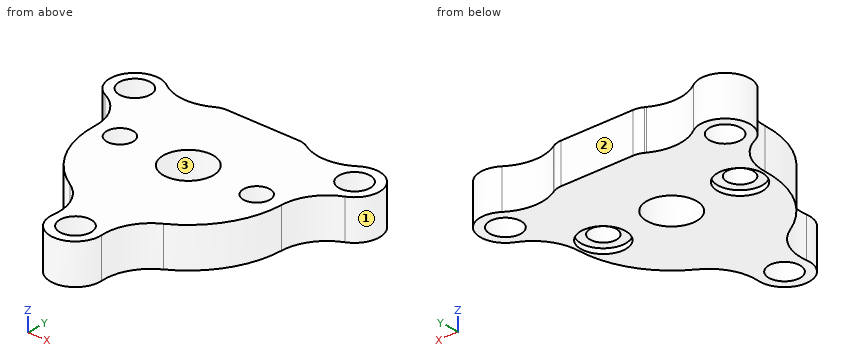
Autodesk Inventor part; units mm, degrees
ref_plane "YZ Plane" through (0, 0, 0) normal (1, 0, 0) x (0, 1, 0)
ref_plane "XZ Plane" through (0, 0, 0) normal (0, 1, 0) x (-1, 0, 0)
ref_plane "XY Plane" through (0, 0, 0) normal (0, 0, 1) x (1, 0, 0)
sketch "Sketch1" plane through (0, 0, 0) normal (0, 0, 1) x (1, 0, 0)
  circle A0 centre (0, 0) radius 20.7359 construction
  line L0 (0, 0) -> (-17.9578, 10.368) construction
  arc A1 (-19.6042, 6.7568) -> (-15.6537, 13.5993) centre (-17.9578, 10.368) ccw construction
  arc A2 (-7.603, 13.208) -> (-15.24, -0.0196) centre (0, 0) ccw construction
  arc A3 (-15.24, -0.0196) -> (-19.6042, 6.7568) centre (-22.698, -0.0292) ccw
  arc A4 (-15.6537, 13.5993) -> (-7.603, 13.208) centre (-11.3237, 19.6716) ccw
  line L1 (0, 0) -> (-20.7359, 0) construction
  arc A5 (-15.6537, 13.5993) -> (-19.6042, 6.7568) centre (-17.9578, 10.368) ccw
  arc A6 (-15.24, -0.0196) -> (-7.637, -13.1884) centre (0, 0) ccw
  arc A7 (7.637, -13.1884) -> (3.9505, -20.3561) centre (11.3743, -19.6424) ccw
  arc A8 (-3.9505, -20.3561) -> (-7.637, -13.1884) centre (-11.3743, -19.6424) ccw
  arc A9 (-3.9505, -20.3561) -> (3.9505, -20.3561) centre (0, -20.7359) ccw
  arc A10 (7.603, 13.208) -> (15.6537, 13.5993) centre (11.3237, 19.6716) ccw
  arc A11 (19.6042, 6.7568) -> (15.24, -0.0196) centre (22.698, -0.0292) ccw
  arc A12 (19.6042, 6.7568) -> (15.6537, 13.5993) centre (17.9578, 10.368) ccw
  arc A13 (7.603, 13.208) -> (6.643, 13.716) centre (0, 0) ccw
  arc A14 (7.637, -13.1884) -> (15.24, -0.0196) centre (0, 0) ccw
  arc A15 (-7.637, -13.1884) -> (7.637, -13.1884) centre (0, 0) ccw construction
  arc A16 (15.24, -0.0196) -> (7.603, 13.208) centre (0, 0) ccw construction
  circle A17 centre (0, 0) radius 3.9688
  circle A18 centre (0, 0) radius 11.176 construction
  line L2 (0, -20.7359) -> (0, 0) construction
  line L3 (0, 0) -> (11.176, 0) construction
  line L4 (-6.643, 13.716) -> (6.643, 13.716)
  arc A19 (-6.643, 13.716) -> (-7.603, 13.208) centre (0, 0) ccw
  arc A20 (6.643, 13.716) -> (-6.643, 13.716) centre (0, 0) ccw construction
  point P0 (-11.176, 0)
  dimension "d0" = 41.4719
  dimension "d3" = 7.9375
  dimension "d5" = 30
  dimension "d9" = 360
  dimension "d20" = 7.9375
  dimension "d21" = 22.352
  dimension "d22" = 15.24
  dimension "d23" = 13.716
extrude "Extrusion1" add sketch "Sketch1" along normal blind 6.35
hole "Hole1" at (-17.9578, 10.368, 0) at (17.9578, 10.368, 0) at (0, -20.7359, 0) direction (0, 0, 1) diameter 4.9784 end through all
hole "Hole2" at (-11.176, 0, 0) at (11.176, 0, 0) direction (0, 0, 1) diameter 4.2164 end through all
fillet "Fillet1" radius 3.175 2 edges at (-6.643, 13.716, 3.175) (6.643, 13.716, 3.175)
sketch "Sketch2" plane through (0, 0, 0) normal (0, 0, -1) x (-1, 0, 0)
  circle A0 centre (11.176, 0) radius 2.1082
  circle A1 centre (-11.176, 0) radius 2.1082
  circle A2 centre (-11.176, 0) radius 3.5719
  circle A3 centre (11.176, 0) radius 3.5719
  dimension "d32" = 7.1437
  dimension "d33" = 7.1437
extrude "Extrusion2" cut sketch "Sketch2" against normal blind 0.7937
properties part number "Pnuematic Plate" material "Aluminum 6061"
Design review of the part built by this model. Coordinates are the model's own, in mm. Face numbers are marked on the shaded views. Give positions to 0.01 mm unless a question says otherwise; leave off trailing zeros. Order: outer loops, then holes, each group sorted by start corner. A loop starts at its lowest first (then second) coordinate and runs counter-clockwise, first axis right, second up.
1. Add section D-D, the plane x = 14. State the section outline as (y, z) points.
Solution:
outline: (-6.02, 0) - (-2.19, 0) - (-2.19, 0.79) - (2.19, 0.79) - (2.19, 0) - (12.71, 0) - (12.71, 6.35) - (-6.02, 6.35) - close
2. Mouldability with a two-part tool opening along Y and no side actions: class the marked faces 1, 2 and 3 as +Y half, -Y half, draft (parallel to the pull), parting line (faces both ways), or undercut.
Solution:
face 1: parting line
face 2: +Y half
face 3: undercut
3. For pin 1 Ø5.5 at (x, y) = (11.176, 0) entering from +Z; pin 2 Ø1.9 at (x, z) = (-1, 4) entering from +Y; pin 3 Ø1.5 at (y, z) = (-20.5, 2) entering from -X; pin 4 Ø3 at (y, z) = (-1, 2.5) entering from +X, all flat-tipped, find the tip position at first contact; note any pin that passes through.
Solution:
pin 1: stops at z = 6.35
pin 2: stops at y = 13.72
pin 3: stops at x = -3.97
pin 4: stops at x = 15.26
4. Add section C-C, the plane y = -4.5. State the section outline as (x, z) points.
Solution:
outline: (-14.56, 0) - (14.56, 0) - (14.56, 6.35) - (-14.56, 6.35) - close
5. To check wall thickness, follow L1, parallel to Y at x = 0.5, z = 2; L2, parallel to Y at x = 11, z = 5; L3, parallel to Y at x = -13, z = 0.75. State the ranges of each line that lie inside material, in increasing order.
Solution:
L1: y = -24.67 to -23.17, -18.3 to -3.94, 3.94 to 13.72
L2: y = -10.55 to -2.1, 2.1 to 12.22
L3: y = -7.95 to -3.07, 3.07 to 12.4
6. Add section A-A, the plane x = 0. State the section outline as (y, z) points.
Solution:
outline: (-24.7, 0) - (-23.23, 0) - (-23.23, 6.35) - (-24.7, 6.35) - close; (-18.25, 0) - (-3.97, 0) - (-3.97, 6.35) - (-18.25, 6.35) - close; (3.97, 0) - (13.72, 0) - (13.72, 6.35) - (3.97, 6.35) - close
7. Add section B-B, the plane z = 3.5. State how many separate pieces and enclosed holes the cut face has, then the cut area to 3 significant figures.
Solution:
separate pieces: 1
enclosed holes: 6
area: 810 mm2
